from build123d import *

# Parameters (mm, degrees)
F0_W     = 2.4047140032
F0_H     = 16.4
F0_W_2   = 3
F0_H_2   = 7.5
F0_W_3   = 1.5
F1_DEPTH = 4
F2_DEPTH = 19
F3_R     = 7.49999
F4_R     = 2.5
F5_DEPTH = 29.9057140032
F6_SIZE  = 2.5
F7_R     = 2.5


# Not quite as in the source:
# - a fillet or chamfer is up to 0.001 mm smaller than in the source, because OpenCascade refuses the exact size
# - a feature names something its author has since deleted; it is built from what else it names


with BuildPart() as f1:
    # F0 (on Top) → F1 (new body)
    with BuildSketch(Plane.XY):
        Polygon((-5.6430239742, 11), (-22.4047140032, 11), (-22.4047140032, -11), (22.4047140032, -11), (22.4047140032, 11), (5.6430239742, 11), (0, 11), align=None)
        with Locations((-18.7023570016, 0)):
            Rectangle(F0_W, F0_H, mode=Mode.SUBTRACT)
        Polygon((-1.5, 7.5), (0, 7.5), (1.5, 7.5), (4.5, 7.5), (7.5, 7.5), (7.5, -7.5), (4.5, -7.5), (4.5, 0), (1.5, 0), (1.5, -7.5), (-1.5, -7.5), (-1.5, 0), (-4.5, 0), (-4.5, -7.5), (-7.5, -7.5), (-7.5, 7.5), (-4.5, 7.5), align=None, mode=Mode.SUBTRACT)
        with Locations((18.7023570016, 0)):
            Rectangle(F0_W, F0_H, mode=Mode.SUBTRACT)
        Polygon((-4.5, 0), (-4.5, 7.5), (-7.5, 7.5), (-7.5, -7.5), (-4.5, -7.5), align=None)
        with Locations((-3, 3.75)):
            Rectangle(F0_W_2, F0_H_2)
        with Locations((-0.75, 3.75)):
            Rectangle(F0_W_3, F0_H_2)
        with Locations((0.75, 3.75)):
            Rectangle(F0_W_3, F0_H_2)
        Polygon((1.5, 0), (0, 0), (-1.5, 0), (-1.5, -7.5), (1.5, -7.5), align=None)
        with Locations((3, 3.75)):
            Rectangle(F0_W_2, F0_H_2)
        Polygon((7.5, 7.5), (4.5, 7.5), (4.5, 0), (4.5, -7.5), (7.5, -7.5), align=None)
    extrude(amount=F1_DEPTH)

    # F0 (on Top) → F2 (join)
    with BuildSketch(Plane.XY):
        Polygon((-4.5, 0), (-4.5, 7.5), (-7.5, 7.5), (-7.5, -7.5), (-4.5, -7.5), align=None)
        with Locations((-0.75, 3.75)):
            Rectangle(F0_W_3, F0_H_2)
        with Locations((0.75, 3.75)):
            Rectangle(F0_W_3, F0_H_2)
        Polygon((1.5, 0), (0, 0), (-1.5, 0), (-1.5, -7.5), (1.5, -7.5), align=None)
        Polygon((7.5, 7.5), (4.5, 7.5), (4.5, 0), (4.5, -7.5), (7.5, -7.5), align=None)
    extrude(amount=F2_DEPTH)

    # F3 (radius 7.5 in the source; OpenCascade refuses exactly that, so slightly less here)
    f3_edges = [f1.edges().sort_by_distance(p)[0] for p in [
        (-6, -7.5, 19),
        (0, -7.5, 19),
        (6, -7.5, 19),
        (6, 7.5, 19),
        (0, 7.5, 19),
        (-6, 7.5, 19),
    ]]
    fillet(f3_edges, radius=F3_R)

    # F4 (on face) → F5 (cut, through all)
    with BuildSketch(Plane(origin=(-7.5, 0, 0), x_dir=(0, -1, 0), z_dir=(-1, 0, 0))):
        with Locations((0, 11.5)):
            Circle(F4_R)
    extrude(amount=-F5_DEPTH, mode=Mode.SUBTRACT)

    # F6
    f6_edges = [f1.edges().sort_by_distance(p)[0] for p in [
        (-6, 7.5, 4),
        (0, 7.5, 4),
        (6, 7.5, 4),
        (-6, -7.5, 4),
        (0, -7.5, 4),
        (6, -7.5, 4),
    ]]
    chamfer(f6_edges, length=F6_SIZE)

    # F7
    f7_edges = [f1.edges().sort_by_distance(p)[0] for p in [
        (-22.404714, 11, 2),
        (-22.404714, -11, 2),
        (22.404714, -11, 2),
        (22.404714, 11, 2),
    ]]
    fillet(f7_edges, radius=F7_R)


solid = f1.part
Check sheet for the modelled part. Datum: model origin and axes. Units: mm. A direction names the side the tool comes from. Round coordinates to 2 decimals unless told otherwise and drop trailing zeros. Order: outer loops, then holes, each group sorted by start corner. A loop starts at its lowest first (then second) coordinate and runs counter-clockwise, first axis right, second up. Notation, with made-up numbers: M 51.5,-26.75 L 71.5,-26.75 A8 ccw 71.5,-14.75 Z; hole C 57,3 d3. An arc over 180 degrees is marked long. One line per item, written item: value. Start each with the question number.
1. Gauge pin test, flat ends, axial feed: P1, Ø1.5, axis at x = -6, z = 9, coming from the +Y side; P2, Ø1.5, axis at x = -6, z = 8.5, coming from the -Y side; P3, Ø1, axis at y = 1, z = 9.5, coming from the +X side; P4, Ø4.5, axis at y = 0, z = 11.5, coming from the +X side. Record the tip position at first contact, or that the pin passes through.
2. Section check A-A on z = 5.5. Enter the section's corners in (x, y), and give its area (3 significant figures).
3. Section check D-D on y = -6.25. Enter the section's corners in (x, z), and give its area (3 significant figures).
4. Section check B-B on z = 10. Enter the section's corners in (x, y).
5. Release check for a two-part mould opening along Y. For faces 4 (the flat face through (-6, -9, 5)), 5 (the flat face through (19, 8.2, 2)), 6 (the flat face through (-1.5, -2.1, 9.7)) record: released by +Y, released by -Y, zero draft, split by the parting line, or undercut.
6. Scan lines: line 1 along X through (y, z) = (-5.75, 14.5); line 2 along X through (y, z) = (-1.5, 1.25); line 3 along Z through (x, y) = (-6.65, 0). Record each from-to range of solid material in increasing order.
7. Access from +Z, -Z, +X, -X, +Y, -Y to the whole of each face (thin tool, end or side, straight path). Record for faces 1 (the flat face through (17.5, 0, 2)), 2 (the flat face through (6, 7.5, 9)), 3 (the flat face through (6, -7.5, 9)).
Results found:
1. P1: y = 7.5
1. P2: y = -7.5
1. P3: x = 7.5
1. P4: through
2. outline: M -7.5,-8.5 L -4.5,-8.5 L -4.5,8.5 L -7.5,8.5 Z; M -1.5,-8.5 L 1.5,-8.5 L 1.5,8.5 L -1.5,8.5 Z; M 4.5,-8.5 L 7.5,-8.5 L 7.5,8.5 L 4.5,8.5 Z
2. area: 153 mm^2
3. outline: M -22.4,0 L -19.9,0 L -19.9,4 L -22.4,4 Z; M -17.5,0 L 17.5,0 L 17.5,4 L 7.5,4 L 7.5,15.65 L 4.5,15.65 L 4.5,4 L 1.5,4 L 1.5,15.65 L -1.5,15.65 L -1.5,4 L -4.5,4 L -4.5,15.65 L -7.5,15.65 L -7.5,4 L -17.5,4 Z; M 19.9,0 L 22.4,0 L 22.4,4 L 19.9,4 Z
3. area: 265 mm^2
4. outline: M -7.5,-7.5 L -4.5,-7.5 L -4.5,-2 L -7.5,-2 Z; M -7.5,2 L -4.5,2 L -4.5,7.5 L -7.5,7.5 Z; M -1.5,-7.5 L 1.5,-7.5 L 1.5,-2 L -1.5,-2 Z; M -1.5,2 L 1.5,2 L 1.5,7.5 L -1.5,7.5 Z; M 4.5,-7.5 L 7.5,-7.5 L 7.5,-2 L 4.5,-2 Z; M 4.5,2 L 7.5,2 L 7.5,7.5 L 4.5,7.5 Z
5. face 4: released by -Y
5. face 5: undercut
5. face 6: zero draft
6. line 1: -7.5 to -4.5, -1.5 to 1.5, 4.5 to 7.5
6. line 2: -22.4 to -19.9, -17.5 to 17.5, 19.9 to 22.4
6. line 3: 0 to 9, 14 to 19
7. face 1: +Z, -Z
7. face 2: +Z, +X, -X, +Y
7. face 3: +Z, +X, -X, -Y
